CAD build for the part. Positions are in the model's coordinates, mm. Face numbers are marked on the shaded views. A direction names the side the tool comes from. Round coordinates to 2 decimals unless told otherwise and drop trailing zeros. Write each loop counter-clockwise with the first axis right and the second up, starting at its lowest first coordinate (ties: lowest second). Pieces come first, ordered by that corner, then holes. Notation, with made-up numbers: (56.25, 71) - (85.25, 71) arc R28 cw to (85.25, 91) - close; hole circle Ø3 at (22.5, 35). An arc over 180 degrees is marked (long way). Put each result on its own line as item: value. Start each with the question number.
Item 1: Drill centre lines: line 1 (X direction, y = 2.5, z = -5.5); line 2 (Z direction, x = 4, y = -0.5); line 3 (Z direction, x = -16, y = -4.25). Where is each one in solid material? Low to high. Write a range as from..to.
Item 2: Pin check, flat tips, straight feed: pin 1 Ø5 at (x, y) = (-9.5, 6.5) entering from -Z; pin 2 Ø8 at (x, z) = (-15.5, -4.5) entering from -Y; pin 3 Ø1.5 at (x, z) = (-16.5, 3) entering from +Y. Stop position of each tip, or through.
Item 3: Cut at D-D (z = 7). Give the cut face in (x, y), and give its area (3 significant figures).
Item 4: Cut at C-C (x = -26). Give the cut face in (y, z), and give its area (3 significant figures).
Item 5: Cut at A-A (y = 0). Give the cut face in (x, z).
Item 6: 3-axis set-ups, long thin cutter, end or side, ignore diameter. For the marked faces 1, 2 and 3: which of +Z, -Z, +X, -X, +Y, -Y reach the whole face in a straight line?
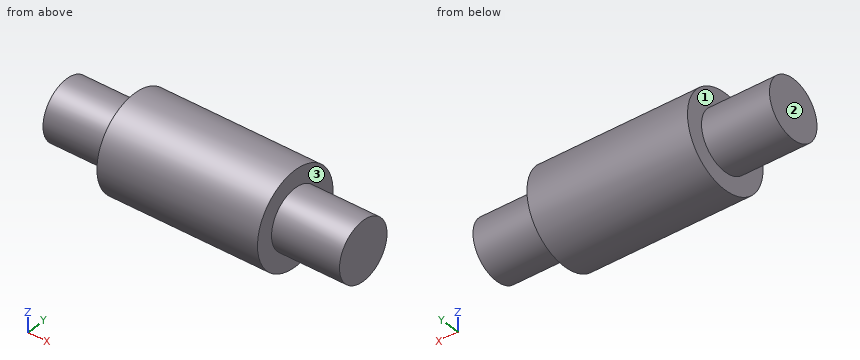
```python
from build123d import *


with BuildPart() as part:
    # CV_Western_4M Sketch → CV_Western_4M (revolve)
    with BuildSketch(Plane.XY, mode=Mode.PRIVATE) as cv_western_4m_sk:
        Polygon((12.7, 0), (12.7, 5.5), (0, 5.5), (0, 8.75), (-30, 8.75), (-30, 5.5), (-42.7, 5.5), (-42.7, 0), align=None)
    revolve(cv_western_4m_sk.sketch.rotate(Axis((-1000, 0, 0), (1, 0, 0)), 90), axis=Axis((-1000, 0, 0), (1, 0, 0)))


solid = part.part
```
Output values:
1. line 1: -30..0
1. line 2: -5.48..5.48
1. line 3: -7.65..7.65
2. pin 1: z = -7.78
2. pin 2: y = -8.74
2. pin 3: y = 8.46
3. outline: (-30, -5.25) - (0, -5.25) - (0, 5.25) - (-30, 5.25) - close
3. area: 315 mm2
4. outline: circle Ø17.5 at (0, 0)
4. area: 241 mm2
5. outline: (-42.7, -5.5) - (-30, -5.5) - (-30, -8.75) - (0, -8.75) - (0, -5.5) - (12.7, -5.5) - (12.7, 5.5) - (0, 5.5) - (0, 8.75) - (-30, 8.75) - (-30, 5.5) - (-42.7, 5.5) - close
6. face 1: -X
6. face 2: +Z, -Z, -X, +Y, -Y
6. face 3: +X
